Design review of the part built by this model. Coordinates are the model's own, in mm. A direction names the side the tool comes from. Coordinates: 2 decimals unless noted, no trailing zeros. Loops run counter-clockwise (first coordinate to the right, second up) from the corner with the lowest first, then second, coordinate; pieces in that order, holes last. Notation, with made-up numbers: (50.25, 2) - (58.25, 2) arc R19 cw to (58.25, 9) - close; hole circle Ø9 at (48.5, -28). An arc over 180 degrees is marked (long way). Use one line per item in the form item = value. Start each with the question number.
(1) Tool access review of faces 1 (the face through (5.974, 2.021, 17.341)), 2 (the face through (-8.2, 8, -0.2)): name each direction out of +Z, -Z, +X, -X, +Y, -Y from which nothing blocks a thin tool from reaching the whole face with its end or side.
(2) Add section D-D (y = 4.75). State the section outline as (x, z) points.
(3) Add section C-C (z = 19.5). State the section outline as (x, y) points, plus the area to 3 significant figures.
(4) The part is to be moulded in two halves that separate along Z. For faces 3 (the face through (0, 2, -23.75)), 4 (the face through (-4, 4.1, 12.2)), 5 (the face through (-3.905, 6.084, -0.867)), say which applies: pulls with the +Z half, pulls with the -Z half, needs draft (parallel to the pull), parting line crosses it, or undercut.
(5) For L1, parallel to X at y = 3, z = 0; L2, parallel to X at y = 7.5, z = 0; L3, parallel to Y at x = 6, z = 12, list the stretches that pass through material, from the lowest coordinate up.
(6) Clearance check with flat-ended pins moving along their axes: pin 1 Ø10 at (x, z) = (-3, 18) entering from +Y; pin 2 Ø4 at (x, z) = (5.5, 1) entering from -Y; pin 3 Ø2 at (x, y) = (1.5, 6.5) entering from +Z; pin 4 Ø4 at (y, z) = (8, -5) entering from -X. State where each tip first meets the part, or that it passes through.
(7) Add section A-A (x = 0). State the section outline as (y, z) points, plus the area to 3 significant figures.
(8) Add section B-B (y = 1.25). State the section outline as (x, z) points.
```python
from build123d import *

# Parameters (mm, degrees)
SKETCH1_R                = 13.25
SKETCH1_R_2              = 2.6
BOSS_EXTRUDE1_DEPTH      = 4.1
BOSS_EXTRUDE2_DEPTH      = 3.9
BOSS_EXTRUDE2_DEPTH_BACK = 4.1
SKETCH2_R                = 12.5
BOSS_EXTRUDE3_DEPTH      = 4
BOSS_EXTRUDE3_DEPTH_BACK = 3.9
SKETCH3_R                = 8
SKETCH4_R                = 4
CUT_EXTRUDE1_DEPTH       = 30.725830518


with BuildPart() as part:
    # Sketch1 → Boss-Extrude1 (new body)
    # profile 1 of 3: a face of its own
    with BuildSketch(Plane(origin=(0, 0, 0), x_dir=(1, 0, 0), z_dir=(0, 1, 0))):
        Circle(SKETCH1_R)
    # profile 2 of 3: a face of its own
    with BuildSketch(Plane(origin=(0, 0, 0), x_dir=(1, 0, 0), z_dir=(0, 1, 0))):
        with BuildLine():
            Line((7.745966692, 10.75), (4.25, 23.75))
            Line((4.25, 23.75), (-4.25, 23.75))
            Line((-4.25, 23.75), (-7.745966692, 10.75))
            ThreePointArc((-7.745966692, 10.75), (0, 13.25), (7.745966692, 10.75))
        make_face()
        with Locations(Location((0, 18.5, 0), (0, 0, 270))):
            Circle(SKETCH1_R_2, mode=Mode.SUBTRACT)
    # profile 3 of 3: a face of its own
    with BuildSketch(Plane(origin=(0, 0, 0), x_dir=(1, 0, 0), z_dir=(0, 1, 0))):
        with BuildLine():
            Line((4.25, -23.75), (7.745966692, -10.75))
            ThreePointArc((7.745966692, -10.75), (0, -13.25), (-7.745966692, -10.75))
            Line((-7.745966692, -10.75), (-4.25, -23.75))
            Line((-4.25, -23.75), (4.25, -23.75))
        make_face()
        with Locations(Location((0, -18.5, 0), (0, 0, 270))):
            Circle(SKETCH1_R_2, mode=Mode.SUBTRACT)
    extrude(amount=BOSS_EXTRUDE1_DEPTH)

    # Sketch2 → Boss-Extrude2 (add, two sides: drawn at the far end of the back side and taken through both)
    with BuildSketch(Plane(origin=(0, 4.1, 0), x_dir=(1, 0, 0), z_dir=(0, 1, 0)).offset(-BOSS_EXTRUDE2_DEPTH_BACK)):
        with Locations(Location((0, 0, 0), (0, 0, 270))):
            Circle(SKETCH2_R)
    extrude(amount=BOSS_EXTRUDE2_DEPTH + BOSS_EXTRUDE2_DEPTH_BACK)

    # Sketch3 → Boss-Extrude3 (add, two sides: drawn at the far end of the back side and taken through both)
    with BuildSketch(Plane(origin=(0, 8, 0), x_dir=(1, 0, 0), z_dir=(0, 1, 0)).offset(-BOSS_EXTRUDE3_DEPTH_BACK)):
        with Locations(Location((0, 0, 0), (0, 0, 270))):
            Circle(SKETCH3_R)
    extrude(amount=BOSS_EXTRUDE3_DEPTH + BOSS_EXTRUDE3_DEPTH_BACK)

    # Sketch4 → Cut-Extrude1 (cut, through all)
    with BuildSketch(Plane(origin=(0, 12, 0), x_dir=(1, 0, 0), z_dir=(0, 1, 0))):
        with Locations(Location((0, 0, 0), (0, 0, 270))):
            Circle(SKETCH4_R)
    extrude(amount=-CUT_EXTRUDE1_DEPTH, mode=Mode.SUBTRACT)


solid = part.part
```
Computed values:
q1.face_1 = +Z, +X, +Y, -Y
q1.face_2 = +Y
q2.outline = circle Ø25 at (0, 0); hole circle Ø8 at (0, 0)
q3.outline = (-5.39, 0) - (-2.4, 0) - (-2.4, 4.1) - (-5.39, 4.1) - close; (2.4, 0) - (5.39, 0) - (5.39, 4.1) - (2.4, 4.1) - close
q3.area = 24.5 mm^2
q4.face_3 = pulls with the -Z half
q4.face_4 = needs draft
q4.face_5 = undercut
q5.L1 = -13.25 to -4, 4 to 13.25
q5.L2 = -12.5 to -4, 4 to 12.5
q5.L3 = 0 to 4.1
q6.pin_1 = 4.1
q6.pin_2 = 0
q6.pin_3 = 12.49
q6.pin_4 = -12.13
q7.outline = (0, -23.75) - (4.1, -23.75) - (4.1, -21.1) - (0, -21.1) - close; (0, -15.9) - (4.1, -15.9) - (4.1, -12.5) - (8, -12.5) - (8, -8) - (12, -8) - (12, -4) - (0, -4) - close; (0, 4) - (12, 4) - (12, 8) - (8, 8) - (8, 12.5) - (4.1, 12.5) - (4.1, 15.9) - (0, 15.9) - close; (0, 21.1) - (4.1, 21.1) - (4.1, 23.75) - (0, 23.75) - close
q7.area = 218 mm^2
q8.outline = (-7.75, -10.75) - (-4.25, -23.75) - (4.25, -23.75) - (7.75, -10.75) arc R13.25 ccw to (7.75, 10.75) - (4.25, 23.75) - (-4.25, 23.75) - (-7.75, 10.75) arc R13.25 ccw to start; hole circle Ø8 at (0, 0); hole circle Ø5.2 at (0, -18.5); hole circle Ø5.2 at (0, 18.5)
